from build123d import *

# Parameters (mm, degrees)
SKETCH1_W                = 39.69
SKETCH1_H                = 3.175
BOSS_EXTRUDE2_DEPTH      = 12.7
CUT_EXTRUDE1_DEPTH       = 12.7
BOSS_EXTRUDE3_DEPTH      = 1.5875
BOSS_EXTRUDE3_DEPTH_BACK = 1.5875
SKETCH5_W                = 5
SKETCH5_H                = 12.7
SKETCH6_W                = 49.69
SKETCH6_H                = 5
BOSS_EXTRUDE4_DEPTH      = 3.175
CUT_EXTRUDE2_DEPTH       = 3.175
SKETCH8_W                = 49.69
SKETCH8_H                = 5
BOSS_EXTRUDE5_DEPTH      = 3.175


with BuildPart() as part:
    # Sketch1 → Boss-Extrude2 (new body)
    with BuildSketch(Plane(origin=(0, 0, 0), x_dir=(1, 0, 0), z_dir=(0, 1, 0))):
        Rectangle(SKETCH1_W, SKETCH1_H)
    extrude(amount=BOSS_EXTRUDE2_DEPTH)

    # Sketch3 → Cut-Extrude1 (cut)
    with BuildSketch(Plane.XY.offset(1.5875)):
        with BuildLine():
            Line((-11, 12.7), (11, 12.7))
            ThreePointArc((11, 12.7), (0, 1.7), (-11, 12.7))
        make_face()
    extrude(amount=-CUT_EXTRUDE1_DEPTH, mode=Mode.SUBTRACT)

    # Sketch5 → Boss-Extrude3 (add, two sides: drawn at the far end of the back side and taken through both)
    with BuildSketch(Plane.XY.offset(-BOSS_EXTRUDE3_DEPTH_BACK)):
        with Locations((22.345, 6.35)):
            Rectangle(SKETCH5_W, SKETCH5_H)
        with Locations((-22.345, 6.35)):
            Rectangle(SKETCH5_W, SKETCH5_H)
    extrude(amount=BOSS_EXTRUDE3_DEPTH + BOSS_EXTRUDE3_DEPTH_BACK)

    # Sketch6 → Boss-Extrude4 (add)
    with BuildSketch(Plane.XY.offset(1.5875)):
        with Locations((0, -2.5)):
            Rectangle(SKETCH6_W, SKETCH6_H)
    extrude(amount=-BOSS_EXTRUDE4_DEPTH)

    # Sketch7 → Cut-Extrude2 (cut)
    with BuildSketch(Plane.XY.offset(1.5875)):
        with BuildLine():
            ThreePointArc((11, 12.7), (0, 1.7), (-11, 12.7))
            Line((-11, 12.7), (-13, 12.7))
            ThreePointArc((-13, 12.7), (0, -0.3), (13, 12.7))
            Line((13, 12.7), (11, 12.7))
        make_face()
    extrude(amount=-CUT_EXTRUDE2_DEPTH, mode=Mode.SUBTRACT)

    # Sketch8 → Boss-Extrude5 (add)
    with BuildSketch(Plane.XY.offset(1.5875)):
        with Locations((0, -7.5)):
            Rectangle(SKETCH8_W, SKETCH8_H)
    extrude(amount=-BOSS_EXTRUDE5_DEPTH)


solid = part.part
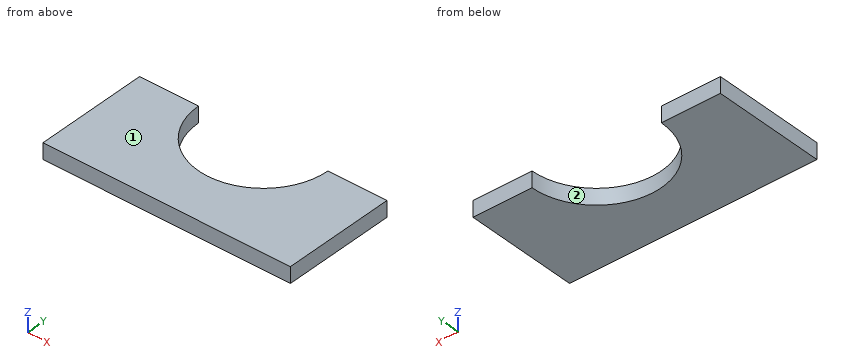
Geometry: final body of the model. Coordinates: model frame, mm. Face numbers are marked on the shaded views. Give positions to 0.01 mm unless a question says otherwise; leave off trailing zeros. Write each loop counter-clockwise with the first axis right and the second up, starting at its lowest first coordinate (ties: lowest second). Pieces come first, ordered by that corner, then holes.
(1) Cut plane B-B, the plane z = 0.3. Return loops of the section in (x, y) (3 decimals).
(2) Mould query, pull axis X, two halves, no side actions, for the marked faces 1 and 2. Classes: released by +X, released by -X, zero draft, split by the parting line, or undercut.
(3) Ray query, line 1 (Y direction, x = 0.5, z = 0); line 2 (X direction, y = 4.75, z = 0.1) (3 decimals); line 3 (X direction, y = 3, z = -0.8) (3 decimals). Return the intervals inside material, ascending.
(4) Cut plane D-D, the plane y = 11. Return loops of the section in (x, z) (1 decimal).
(5) Cut plane C-C, the plane x = 0. Return loops of the section in (y, z), then the cut area to 3 significant figures.
(6) Cut plane A-A, the plane y = 1.5. Return loops of the section in (x, z) (1 decimal).
(7) First-contact query: P1, Ø12, axis at x = 9.5, y = 5, coming from the -Z side. Flat tip, straight axial feed; report the tip coordinate or a pass-through.
Values follow:
1. outline: (-24.845, -10) - (24.845, -10) - (24.845, 12.7) - (13, 12.7) arc R13 cw to (-13, 12.7) - (-24.845, 12.7) - close
2. face 1: zero draft
2. face 2: undercut
3. line 1: y = -10 to -0.29
3. line 2: x = -24.845 to -10.286, 10.286 to 24.845
3. line 3: x = -24.845 to -8.655, 8.655 to 24.845
4. outline: (-24.8, -1.6) - (-12.9, -1.6) - (-12.9, 1.6) - (-24.8, 1.6) - close; (12.9, -1.6) - (24.8, -1.6) - (24.8, 1.6) - (12.9, 1.6) - close
5. outline: (-10, -1.59) - (-0.3, -1.59) - (-0.3, 1.59) - (-10, 1.59) - close
5. area: 30.8 mm2
6. outline: (-24.8, -1.6) - (-6.6, -1.6) - (-6.6, 1.6) - (-24.8, 1.6) - close; (6.6, -1.6) - (24.8, -1.6) - (24.8, 1.6) - (6.6, 1.6) - close
7. P1: stops at z = -1.59
